from build123d import *
from OCP.BRepFilletAPI import BRepFilletAPI_MakeChamfer

# Parameters (mm, degrees)
SKETCH_1_W               = 126.5
SKETCH_1_H               = 82.5
SKETCH_1_W_2             = 28
SKETCH_1_H_2             = 28
EXTRUDE_1_DEPTH          = 8
SKETCH_2_W               = 126.5
SKETCH_2_H               = 23.75
EXTRUDE_2_DEPTH          = 0.3
CHAMFER_1_SIZE           = 1
CHAMFER_1_SIZE2          = 11.430052303
FILLET_1_R               = 2
FILLET_2_R               = 1
CUT_EXTRUDE_1_DEPTH      = 76.935005103
CUT_EXTRUDE_1_DEPTH_BACK = 76.935005103
SKETCH_3_R               = 2.1
CHAMFER_2_SIZE           = 8.342275148
CHAMFER_2_SIZE_2         = 7
CHAMFER_3_SIZE2          = 8
CHAMFER_3_SIZE           = 9.534028741


with BuildPart() as part:
    # Эскиз1 → Бобышка-Вытянуть1 (new body)
    with BuildSketch(Plane(origin=(0, 0, 0), x_dir=(1, 0, 0), z_dir=(0, 1, 0))):
        Rectangle(SKETCH_1_W, SKETCH_1_H)
        Rectangle(SKETCH_1_W_2, SKETCH_1_H_2, mode=Mode.SUBTRACT)
    extrude(amount=EXTRUDE_1_DEPTH)

    # Эскиз2 → Бобышка-Вытянуть2 (add)
    with BuildSketch(Plane(origin=(0, 8, 0), x_dir=(1, 0, 0), z_dir=(0, 1, 0))):
        with Locations((0, 29.375)):
            Rectangle(SKETCH_2_W, SKETCH_2_H)
        with Locations((0, -29.375)):
            Rectangle(SKETCH_2_W, SKETCH_2_H)
    extrude(amount=EXTRUDE_2_DEPTH)

    # Фаска1: one chamfer whose edges measure the first distance from different faces: ONE call of the kernel's chamfer builder (chamfer() names one face for all edges)
    chamfer_1_edges_1 = [part.edges().sort_by_distance(p)[0] for p in [
        (-63.25, 8, 0),
    ]]
    chamfer_1_side_1 = [part.faces().sort_by_distance(p)[0] for p in [
        (-63.25, 4.087708565, 0),
    ]]
    chamfer_1_edges_2 = [part.edges().sort_by_distance(p)[0] for p in [
        (63.25, 8, 0),
    ]]
    chamfer_1_side_2 = [part.faces().sort_by_distance(p)[0] for p in [
        (63.25, 4.087708565, 0),
    ]]
    chamfer_1 = BRepFilletAPI_MakeChamfer(part.part.solid().wrapped)
    for e in chamfer_1_edges_1:
        chamfer_1.Add(CHAMFER_1_SIZE, CHAMFER_1_SIZE2, e.wrapped, chamfer_1_side_1[0].wrapped)  # the first distance lies on this face
    for e in chamfer_1_edges_2:
        chamfer_1.Add(CHAMFER_1_SIZE, CHAMFER_1_SIZE2, e.wrapped, chamfer_1_side_2[0].wrapped)  # the first distance lies on this face
    add(Compound.cast(chamfer_1.Shape()), mode=Mode.REPLACE)

    # Скругление1
    fillet_1_edges = [part.edges().sort_by_distance(p)[0] for p in [
        (63.25, 7, 0),
        (-63.25, 7, 0),
    ]]
    fillet(fillet_1_edges, radius=FILLET_1_R)

    # Скругление2
    fillet_2_edges = [part.edges().sort_by_distance(p)[0] for p in [
        (-14, 8, 0),
        (14, 8, 0),
    ]]
    fillet(fillet_2_edges, radius=FILLET_2_R)

    # Эскиз3 → Вырез-Вытянуть1 (cut, two sides: drawn at the far end of the back side and taken through both)
    with BuildSketch(Plane(origin=(0, 8, 0), x_dir=(1, 0, 0), z_dir=(0, 1, 0)).offset(-CUT_EXTRUDE_1_DEPTH_BACK)):
        with Locations(Location((-40, 30, 0), (0, 0, 270))):
            Circle(SKETCH_3_R)
        with Locations(Location((40, 30, 0), (0, 0, 270))):
            Circle(SKETCH_3_R)
        with Locations(Location((-40, -30, 0), (0, 0, 270))):
            Circle(SKETCH_3_R)
        with Locations(Location((40, -30, 0), (0, 0, 270))):
            Circle(SKETCH_3_R)
    extrude(amount=CUT_EXTRUDE_1_DEPTH + CUT_EXTRUDE_1_DEPTH_BACK, mode=Mode.SUBTRACT)

    # Фаска2
    chamfer_2_edges_1 = [part.edges().sort_by_distance(p)[0] for p in [
        (14, 0, 0),
    ]]
    chamfer_2_side_1 = [part.faces().sort_by_distance(p)[0] for p in [
        (14.14, 0, 0),
    ]]
    chamfer_2_edges_2 = [part.edges().sort_by_distance(p)[0] for p in [
        (-14, 0, 0),
    ]]
    chamfer_2_side_2 = [part.faces().sort_by_distance(p)[0] for p in [
        (-14.14, 0, 0),
    ]]
    chamfer_2 = BRepFilletAPI_MakeChamfer(part.part.solid().wrapped)
    for e in chamfer_2_edges_1:
        chamfer_2.Add(CHAMFER_2_SIZE - 0.0001, CHAMFER_2_SIZE_2 - 0.0001, e.wrapped, chamfer_2_side_1[0].wrapped)
    for e in chamfer_2_edges_2:
        chamfer_2.Add(CHAMFER_2_SIZE - 0.0001, CHAMFER_2_SIZE_2 - 0.0001, e.wrapped, chamfer_2_side_2[0].wrapped)
    add(Compound.cast(chamfer_2.Shape()), mode=Mode.REPLACE)  # a hair under: the kernel refuses the full size

    # Фаска3
    chamfer_3_edges = [part.edges().sort_by_distance(p)[0] for p in [
        (0, 0, -14),
    ]]
    chamfer_3_side = [part.faces().sort_by_distance(p)[0] for p in [
        (0, 0, -14.16),
    ]]
    chamfer(chamfer_3_edges, length=CHAMFER_3_SIZE - 0.0001, length2=CHAMFER_3_SIZE2 - 0.0001, reference=chamfer_3_side[0])  # a hair under: the kernel refuses the full size
    chamfer_3_2_edges = [part.edges().sort_by_distance(p)[0] for p in [
        (0, 0, 14),
    ]]
    chamfer_3_2_side = [part.faces().sort_by_distance(p)[0] for p in [
        (0, 0, 14.16),
    ]]
    chamfer(chamfer_3_2_edges, length=CHAMFER_3_SIZE - 0.0001, length2=CHAMFER_3_SIZE2 - 0.0001, reference=chamfer_3_2_side[0])  # a hair under: the kernel refuses the full size


solid = part.part
For this review, take the finished solid that the model builds, in its own axes (mm). A direction names the side the tool comes from. Round coordinates to 2 decimals unless told otherwise and drop trailing zeros. Write each loop counter-clockwise with the first axis right and the second up, starting at its lowest first coordinate (ties: lowest second). Pieces come first, ordered by that corner, then holes. Notation, with made-up numbers: (71, 20.5) - (91, 20.5) arc R13 ccw to (91, 38.5) - close; hole circle Ø3 at (51, 13.5). An arc over 180 degrees is marked (long way). Write item = value, one per line. Start each with the question number.
1. Wall thickness on L1, parallel to Z at x = 40, y = 2.5; L2, parallel to X at y = 4, z = 30; L3, parallel to Z at x = 45, y = 8.25: over which ranges is each line inside the solid? List them lowest first.
2. Draft analysis for pull direction Z (two halves, no side actions). For faces 1 (the face through (-41.278, 4.092, -31.666)), 2 (the face through (56.555, 7.586, 0.245)), 3 (the face through (-1, 4, -41.25)), 4 (the face through (-1, 4, 41.25)), state which applies: released by +Z, released by -Z, zero draft, split by the parting line, or undercut.
3. Consider section A-A on x = -40. State the section outline as (y, z) points, plus the area to 3 significant figures.
4. For pin 1 Ø17.5 at (x, z) = (21, -8) entering from +Y; pin 2 Ø12 at (x, z) = (16, 15) entering from -Y, all flat-tipped, find the tip position at first contact; note any pin that passes through.
5. For faces 5 (the face through (-56.555, 7.586, 0.245)), 6 (the face through (-18.11, 3.55, 0.33)), 7 (the face through (-1, 8, 15)), list the 3-axis set-ups (+Z, -Z, +X, -X, +Y, -Y) from which the entire face can be reached by the end or side of a thin tool; tool diameter is ignored.
6. Consider section C-C on z = 30. State the section outline as (x, y) points.
Evaluation:
q1.L1 = -41.25 to -32.1, -27.9 to 27.9, 32.1 to 41.25
q1.L2 = -63.25 to -42.1, -37.9 to 37.9, 42.1 to 63.25
q1.L3 = -41.25 to -17.5, 17.5 to 41.25
q2.face_1 = undercut
q2.face_2 = undercut
q2.face_3 = released by -Z
q2.face_4 = released by +Z
q3.outline = (0, -41.25) - (8.3, -41.25) - (8.3, -32.1) - (0, -32.1) - close; (0, -27.9) - (8.3, -27.9) - (8.3, -17.5) - (8, -17.5) - (8, 17.5) - (8.3, 17.5) - (8.3, 27.9) - (0, 27.9) - close; (0, 32.1) - (8.3, 32.1) - (8.3, 41.25) - (0, 41.25) - close
q3.area = 605 mm2
q4.pin_1 = 8
q4.pin_2 = 0.29
q5.face_5 = -X, +Y
q5.face_6 = -Y
q5.face_7 = +X, -X, +Y
q6.outline = (-63.25, 0) - (-42.1, 0) - (-42.1, 8.3) - (-63.25, 8.3) - close; (-37.9, 0) - (37.9, 0) - (37.9, 8.3) - (-37.9, 8.3) - close; (42.1, 0) - (63.25, 0) - (63.25, 8.3) - (42.1, 8.3) - close
